The model under review builds one solid part; all positions refer to its coordinate system, in mm. Coordinates: 2 decimals unless noted, no trailing zeros. Order: outer loops, then holes, each group sorted by start corner. A loop starts at its lowest first (then second) coordinate and runs counter-clockwise, first axis right, second up. Notation, with made-up numbers: M -9.5,25 L 41.5,25 A32 cw 41.5,56 Z; hole C 87.5,26.25 d11. An arc over 180 degrees is marked long. Answer as CSV lines item,"result". Start each with the question number.
Q1. Consider section B-B on z = 3.25. Write out the cut boundary in (x, y).
Q2. For P1, Ø0.6, axis at x = 1, y = -7, coming from the +Z side (3 decimals); P2, Ø1, axis at x = -4.5, z = 3.5, coming from the -Y side, all flat-tipped, find the tip position at first contact; note any pin that passes through.
Q3. Consider section A-A on x = -3.75. Write out the cut boundary in (y, z) (3 decimals), and give its area (3 significant figures).
Q4. Wall thickness on L1, parallel to X at y = -6.5, z = 5.1; L2, parallel to Y at x = -0.25, z = 1.55: over which ranges is each line inside the solid? List them lowest first. Write a range as [from, to].
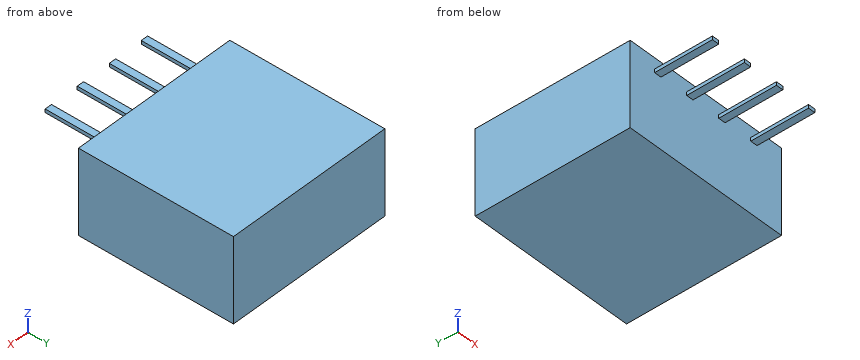
from build123d import *

# Parameters (mm, degrees)
SKETCH1_W           = 12
SKETCH1_H           = 11
BOSS_EXTRUDE1_DEPTH = 6
SKETCH2_W           = 0.5
SKETCH2_H           = 0.25
BOSS_EXTRUDE2_DEPTH = 4.1


with BuildPart() as part:
    # Sketch1 → Boss-Extrude1 (new body)
    with BuildSketch(Plane.XY):
        Rectangle(SKETCH1_W, SKETCH1_H)
    extrude(amount=BOSS_EXTRUDE1_DEPTH)

    # Sketch2 → Boss-Extrude2 (add)
    with BuildSketch(Plane.XZ.offset(5.5)):
        with Locations((1.27, 5.1)):
            Rectangle(SKETCH2_W, SKETCH2_H)
        with Locations((3.81, 5.1)):
            Rectangle(SKETCH2_W, SKETCH2_H)
        with Locations((-1.27, 5.1)):
            Rectangle(SKETCH2_W, SKETCH2_H)
        with Locations((-3.81, 5.1)):
            Rectangle(SKETCH2_W, SKETCH2_H)
    extrude(amount=BOSS_EXTRUDE2_DEPTH)


solid = part.part
Evaluation:
1,outline,"M -6,-5.5 L 6,-5.5 L 6,5.5 L -6,5.5 Z"
2,P1,"stops at z = 5.225"
2,P2,"stops at y = -5.5"
3,outline,"M -9.6,4.975 L -5.5,4.975 L -5.5,0 L 5.5,0 L 5.5,6 L -5.5,6 L -5.5,5.225 L -9.6,5.225 Z"
3,area,"67.0 mm²"
4,L1,"x = [-4.06, -3.56], [-1.52, -1.02], [1.02, 1.52], [3.56, 4.06]"
4,L2,"y = [-5.5, 5.5]"
